Autodesk Inventor part; units mm, degrees
ref_plane "YZ Plane" through (0, 0, 0) normal (1, 0, 0) x (0, 1, 0)
ref_plane "XZ Plane" through (0, 0, 0) normal (0, 1, 0) x (-1, 0, 0)
ref_plane "XY Plane" through (0, 0, 0) normal (0, 0, 1) x (1, 0, 0)
sketch "Sketch1" plane through (0, 0, 0) normal (0, 1, 0) x (-1, 0, 0)
  line L0 (0, 0) -> (45.72, 0)
  line L1 (45.72, 0) -> (45.72, -34.798)
  line L2 (45.72, -34.798) -> (0, -85.09)
  line L3 (0, -85.09) -> (0, 0) construction
  line L4 (0, 0) -> (-45.72, 0)
  line L5 (-45.72, 0) -> (-45.72, -34.798)
  line L6 (-45.72, -34.798) -> (0, -85.09)
  dimension "d0" = 45.72
  dimension "d1" = 85.09
  dimension "d2" = 34.798
extrude "Extrusion1" add sketch "Sketch1" along normal blind 2.921
sketch "Sketch3" plane through (0, 2.921, 0) normal (0, 1, 0) x (1, 0, 0)
  line L0 (-45.72, 0) -> (45.72, 0)
  line L1 (45.72, 0) -> (45.72, 34.798)
  line L2 (-45.72, 0) -> (45.72, 0)
  line L3 (45.72, 0) -> (45.72, 2.921)
  line L4 (45.72, 2.921) -> (-45.72, 2.921)
  line L5 (-45.72, 2.921) -> (-45.72, 0)
  point P0 (0, 0)
  dimension "d5" = 2.921
extrude "Extrusion2" add sketch "Sketch3" along normal blind 17.399
fillet "Fillet1" radius 3.175 1 edges at (0, 1.4605, -85.09)
fillet "Fillet2" radius 3.175 2 edges at (45.72, 1.4605, -34.798) (-45.72, 1.4605, -34.798)
fillet "Fillet3" radius 3.175 1 edges at (0, 2.921, -2.921)
properties part number "SnowBlowerMotorMount"
Read the model definition and answer for the solid it produces. Units are mm, in the model's axes. A direction names the side the tool comes from. Coordinates: 2 decimals unless noted, no trailing zeros. Loops run counter-clockwise (first coordinate to the right, second up) from the corner with the lowest first, then second, coordinate; pieces in that order, holes last.
Q1. The part is cut by section D-D on z = -30. Write down the section's boundary in (x, y).
Q2. The part is cut by section A-A on x = 25.5. Write down the section's boundary in (y, z) (3 decimals).
Q3. Consider probe 1 along Y at (x, z) = (-7, -70); probe 2 along Z at (x, y) = (-39, 9.25); probe 3 along Z at (x, y) = (-5, 1.25). Determine where each line is inside the solid, lowest interval first.
Q4. The part is cut by section C-C on x = -20. Write down the section's boundary in (y, z) (3 decimals).
Q5. Each of these flat-tipped pins is pushed along its axis until it touches: pin 1 Ø6 at (x, z) = (16.5, -58) entering from +Y; pin 2 Ø7 at (x, y) = (-3.5, 13) entering from -Z; pin 3 Ø6 at (y, z) = (7.5, -17) entering from -X; pin 4 Ø4 at (y, z) = (4.5, -54) entering from +X. Where does it stop, or does it pass through?
Q6. Which of the six approach directions +Z, -Z, +X, -X, +Y, -Y give full straight-line access (tool end or side, diameter ignored) to faces 1 (the face through (1, 2.921, -36)), 2 (the face through (-45.5, 1.48, -34.73))?
Q7. The part is cut by section B-B on y = 1.75. Write down the section's boundary in (x, z) (3 decimals).
Results below:
1. outline: (-45.72, 0) - (45.72, 0) - (45.72, 2.92) - (-45.72, 2.92) - close
2. outline: (0, -57.04) - (2.921, -57.04) - (2.921, -6.096) arc R3.175 cw to (6.096, -2.921) - (20.32, -2.921) - (20.32, 0) - (0, 0) - close
3. probe 1: y = 0 to 2.92
3. probe 2: z = -2.92 to 0
3. probe 3: z = -79.59 to 0
4. outline: (0, -63.09) - (2.921, -63.09) - (2.921, -6.096) arc R3.175 cw to (6.096, -2.921) - (20.32, -2.921) - (20.32, 0) - (0, 0) - close
5. pin 1: stops at y = 2.92
5. pin 2: stops at z = -2.92
5. pin 3: passes through
5. pin 4: stops at x = 29.38
6. face 1: -Z, +X, -X, +Y
6. face 2: -Z, -X, +Y, -Y
7. outline: (-45.72, -33.571) arc R3.175 ccw to (-44.894, -35.706) - (-2.349, -82.506) arc R3.175 ccw to (2.349, -82.506) - (44.894, -35.706) arc R3.175 ccw to (45.72, -33.571) - (45.72, 0) - (-45.72, 0) - close
